```python
from build123d import *

# Parameters (mm, degrees)
EXTRUDE_1_DEPTH          = 80
SKETCH_2_W               = 10
SKETCH_2_H               = 3
EXTRUDE_2_DEPTH          = 11.5
SKETCH_3_R               = 2
CUT_EXTRUDE_2_DEPTH      = 81
CUT_EXTRUDE_2_DEPTH_BACK = 1


with BuildPart() as part:
    # 草图1 → 凸台-拉伸1 (new body)
    with BuildSketch(Plane(origin=(0, 0, 0), x_dir=(1, 0, 0), z_dir=(0, 1, 0))):
        Polygon((11.5, 5), (11.5, 8), (-11.5, 8), (-11.5, 5), (-1.5, 5), (-1.5, -5), (-11.5, -5), (-11.5, -8), (11.5, -8), (11.5, -5), (1.5, -5), (1.5, 5), align=None)
    extrude(amount=EXTRUDE_1_DEPTH)

    # 草图2 → 凸台-拉伸2 (add, symmetric)
    with BuildSketch(Plane(origin=(0, 0, 0), x_dir=(0, 0, -1), z_dir=(1, 0, 0))):
        with Locations((0, 1.5)):
            Rectangle(SKETCH_2_W, SKETCH_2_H)
        with Locations((0, 78.5)):
            Rectangle(SKETCH_2_W, SKETCH_2_H)
    extrude(amount=EXTRUDE_2_DEPTH, both=True)

    # 草图3 → 切除-拉伸2 (cut, two sides)
    with BuildSketch(Plane(origin=(0, 0, 0), x_dir=(1, 0, 0), z_dir=(0, 1, 0))) as cut_extrude_2_sk:
        with Locations((6.5, 0)):
            Circle(SKETCH_3_R)
        with Locations((-6.5, 0)):
            Circle(SKETCH_3_R)
    extrude(amount=CUT_EXTRUDE_2_DEPTH, mode=Mode.SUBTRACT)
    extrude(cut_extrude_2_sk.sketch, amount=-CUT_EXTRUDE_2_DEPTH_BACK, mode=Mode.SUBTRACT)


solid = part.part
```
Part model, mm, in its own coordinate system. A direction names the side the tool comes from. Round coordinates to 2 decimals unless told otherwise and drop trailing zeros. Loops run counter-clockwise (first coordinate to the right, second up) from the corner with the lowest first, then second, coordinate; pieces in that order, holes last. Notation, with made-up numbers: (-30, -11.75) -> (10, -11.75) arc R32 cw to (10, 20.25) -> close; hole circle Ø5 at (45.25, 57). An arc over 180 degrees is marked (long way). Use a Markdown table: item, result.
1) Cut at D-D, the plane z = -3.75. List the corners of the cut face in (x, y).
The answers:
| item | result |
|---|---|
| outline | (-11.5, 0) -> (11.5, 0) -> (11.5, 3) -> (1.5, 3) -> (1.5, 77) -> (11.5, 77) -> (11.5, 80) -> (-11.5, 80) -> (-11.5, 77) -> (-1.5, 77) -> (-1.5, 3) -> (-11.5, 3) -> close |
2) Pull direction Y, two halves, no side cores. Call faces 1 (the flat face through (-7, 39, -5)), 2 (the flat face through (0, 80, 0)), 3 (the cylindrical face through (4.9, 1.5, 1.2)): pulls with the +Y half, pulls with the -Y half, needs draft (parallel to the pull), parting line crosses it, or undercut.
The answers:
| item | result |
|---|---|
| face 1 | undercut |
| face 2 | pulls with the +Y half |
| face 3 | needs draft |
3) Drop flat-ended pins along their axis: pin 1 Ø3 at (y, z) = (28, 0) entering from -X; pin 2 Ø8 at (y, z) = (35.5, 1.5) entering from +X. Give the stop position or say it passes through.
The answers:
| item | result |
|---|---|
| pin 1 | stops at x = -1.5 |
| pin 2 | stops at x = 11.5 |
4) Cut at B-B, the plane x = -6.5. List the corners of the cut face in (y, z), and give its area (3 significant figures).
The answers:
| item | result |
|---|---|
| outline | (0, -8) -> (80, -8) -> (80, -2) -> (77, -2) -> (77, -5) -> (3, -5) -> (3, -2) -> (0, -2) -> close; (0, 2) -> (3, 2) -> (3, 5) -> (77, 5) -> (77, 2) -> (80, 2) -> (80, 8) -> (0, 8) -> close |
| area | 516 mm2 |
5) Cut at C-C, the plane y = 12.5. List the corners of the cut face in (x, z).
The answers:
| item | result |
|---|---|
| outline | (-11.5, -8) -> (11.5, -8) -> (11.5, -5) -> (1.5, -5) -> (1.5, 5) -> (11.5, 5) -> (11.5, 8) -> (-11.5, 8) -> (-11.5, 5) -> (-1.5, 5) -> (-1.5, -5) -> (-11.5, -5) -> close |
6) Cut at A-A, the plane z = 0. List the corners of the cut face in (x, y).
The answers:
| item | result |
|---|---|
| outline | (-11.5, 0) -> (-8.5, 0) -> (-8.5, 3) -> (-11.5, 3) -> close; (-11.5, 77) -> (-8.5, 77) -> (-8.5, 80) -> (-11.5, 80) -> close; (-4.5, 0) -> (4.5, 0) -> (4.5, 3) -> (1.5, 3) -> (1.5, 77) -> (4.5, 77) -> (4.5, 80) -> (-4.5, 80) -> (-4.5, 77) -> (-1.5, 77) -> (-1.5, 3) -> (-4.5, 3) -> close; (8.5, 0) -> (11.5, 0) -> (11.5, 3) -> (8.5, 3) -> close; (8.5, 77) -> (11.5, 77) -> (11.5, 80) -> (8.5, 80) -> close |
7) Tool access for faces 4 (the flat face through (0, 39, 8)), 5 (the flat face through (7, 39, 5)), 6 (the flat face through (-1.5, 39, 0)): list every direction of +Z, -Z, +X, -X, +Y, -Y with a clear straight run to the whole face (end or side of a thin tool).
The answers:
| item | result |
|---|---|
| face 4 | +Z, +X, -X, +Y, -Y |
| face 5 | +X |
| face 6 | -X |
8) Probe line 1 (Z direction, x = -6.5, y = 1.55); line 2 (Y direction, x = 4.75, z = 4); line 3 (Z direction, x = -2.5, y = 7.5). List the from-to ranges inside material, lowest first. Write a range as [from, to].
The answers:
| item | result |
|---|---|
| line 1 | z = [-8, -2], [2, 8] |
| line 2 | y = [0, 3], [77, 80] |
| line 3 | z = [-8, -5], [5, 8] |
